from build123d import *

# Parameters (mm, degrees)
SKETCH1_W           = 16
SKETCH1_H           = 16
BOSS_EXTRUDE1_DEPTH = 1.5875
BOSS_EXTRUDE2_DEPTH = 3.625
BOSS_EXTRUDE3_DEPTH = 1.5875
SKETCH5_R           = 0.599365756
BOSS_EXTRUDE6_DEPTH = 50
SKETCH6_R           = 0.881021891
BOSS_EXTRUDE7_DEPTH = 2
BOSS_EXTRUDE8_DEPTH = 4
SKETCH8_R           = 1.431086417
BOSS_EXTRUDE9_DEPTH = 1.75
SKETCH9_R           = 1.026782917
SKETCH9_R_2         = 0.386874667
CUT_EXTRUDE1_DEPTH  = 0.5


with BuildPart() as part:
    # Sketch1 → Boss-Extrude1 (new body)
    with BuildSketch(Plane(origin=(0, 0, 0), x_dir=(1, 0, 0), z_dir=(0, 1, 0))):
        Rectangle(SKETCH1_W, SKETCH1_H)
    extrude(amount=BOSS_EXTRUDE1_DEPTH)

    # Sketch2 → Boss-Extrude2 (add)
    with BuildSketch(Plane(origin=(0, 1.5875, 0), x_dir=(1, 0, 0), z_dir=(0, 1, 0))):
        with BuildLine():
            Line((-6.5, -7.5), (6.5, -7.5))
            ThreePointArc((6.5, -7.5), (7.207106781, -7.207106781), (7.5, -6.5))
            Line((7.5, -6.5), (7.5, 6.5))
            ThreePointArc((7.5, 6.5), (7.207106781, 7.207106781), (6.5, 7.5))
            Line((6.5, 7.5), (-6.5, 7.5))
            ThreePointArc((-6.5, 7.5), (-7.207106781, 7.207106781), (-7.5, 6.5))
            Line((-7.5, 6.5), (-7.5, -6.5))
            ThreePointArc((-7.5, -6.5), (-7.207106781, -7.207106781), (-6.5, -7.5))
        make_face()
    extrude(amount=BOSS_EXTRUDE2_DEPTH)

    # Sketch4 → Boss-Extrude3 (add)
    with BuildSketch(Plane.XZ):
        Polygon((5, 6), (-5, 6), (-6, 5), (-6, -5), (-5, -6), (5, -6), (6, -5), (6, 5), align=None)
    extrude(amount=BOSS_EXTRUDE3_DEPTH)

    # Sketch5 → Boss-Extrude6 (add)
    with BuildSketch(Plane(origin=(6, 0, 0), x_dir=(0, 0, -1), z_dir=(1, 0, 0))):
        with Locations(Location((0, -0.711731406, 0), (0, 0, 180))):
            Circle(SKETCH5_R)
    extrude(amount=BOSS_EXTRUDE6_DEPTH)

    # Sketch6 → Boss-Extrude7 (add)
    with BuildSketch(Plane(origin=(56, 0, 0), x_dir=(0, 0, -1), z_dir=(1, 0, 0))):
        with Locations((0, -0.711731406)):
            Circle(SKETCH6_R)
    extrude(amount=BOSS_EXTRUDE7_DEPTH)

    # Sketch7 → Boss-Extrude8 (add)
    with BuildSketch(Plane(origin=(58, 0, 0), x_dir=(0, 0, -1), z_dir=(1, 0, 0))):
        with BuildLine():
            Line((-0.493950471, 0.22540454), (0.493950471, 0.22540454))
            ThreePointArc((0.493950471, 0.22540454), (1.431086417, -0.711731406), (0.493950471, -1.648867351))
            Line((0.493950471, -1.648867351), (-0.493950471, -1.648867351))
            ThreePointArc((-0.493950471, -1.648867351), (-1.431086417, -0.711731406), (-0.493950471, 0.22540454))
        make_face()
    extrude(amount=BOSS_EXTRUDE8_DEPTH)

    # Sketch8 → Boss-Extrude9 (add)
    with BuildSketch(Plane.XZ.offset(0.711731406)):
        with Locations(Location((60.568913583, 0, 0), (0, 0, 270))):
            Circle(SKETCH8_R)
    extrude(amount=BOSS_EXTRUDE9_DEPTH)

    # Sketch9 → Cut-Extrude1 (cut)
    with BuildSketch(Plane(origin=(0, -2.461731406, 0), x_dir=(-1, 0, 0), z_dir=(0, -1, 0))):
        with Locations(Location((-60.568913583, 0, 0), (0, 0, 90))):
            Circle(SKETCH9_R)
        with Locations(Location((-60.568913583, 0, 0), (0, 0, 90))):
            Circle(SKETCH9_R_2, mode=Mode.SUBTRACT)
    extrude(amount=-CUT_EXTRUDE1_DEPTH, mode=Mode.SUBTRACT)


solid = part.part
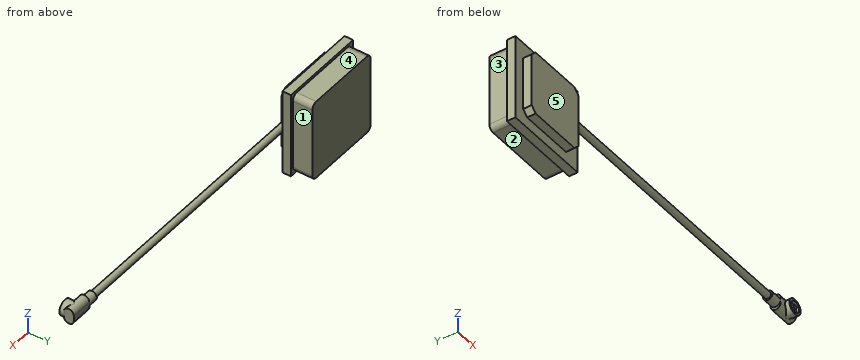
CAD build for the part. Positions are in the model's coordinates, mm. Face numbers are marked on the shaded views. A direction names the side the tool comes from. Coordinates: 2 decimals unless noted, no trailing zeros. Order: outer loops, then holes, each group sorted by start corner. A loop starts at its lowest first (then second) coordinate and runs counter-clockwise, first axis right, second up. Notation, with made-up numbers: (-4, 40) -> (48, 40) arc R15 ccw to (48, 51) -> close; hole circle Ø5 at (54, 37). An arc over 180 degrees is marked (long way). Answer in a Markdown table with one row per item.
1) Which spindle directions (+Z, -Z, +X, -X, +Y, -Y) get a long thin tool onto all of the face, cutting with end or side? Do the marked faces 1, 2, 3, 4 and 5. Say none if no direction does.
Check values:
| item | result |
|---|---|
| face 1 | +Z, -Z, +X, +Y |
| face 2 | -Z, +X, -X, +Y |
| face 3 | +Z, -Z, -X, +Y |
| face 4 | +Z, +X, -X, +Y |
| face 5 | +Z, -Z, -X, -Y |
2) Band-saw the part on B-B (x = 47.5). List the corners of the cut face in (y, z), and give its area (3 significant figures).
Check values:
| item | result |
|---|---|
| outline | circle Ø1.2 at (-0.71, 0) |
| area | 1.13 mm2 |
3) Band-saw the part on A-A (z = 3). List the corners of the cut face in (x, y), and give its area (3 significant figures).
Check values:
| item | result |
|---|---|
| outline | (-8, 0) -> (-6, 0) -> (-6, -1.59) -> (6, -1.59) -> (6, 0) -> (8, 0) -> (8, 1.59) -> (7.5, 1.59) -> (7.5, 5.21) -> (-7.5, 5.21) -> (-7.5, 1.59) -> (-8, 1.59) -> close |
| area | 98.8 mm2 |
4) Drill centre lines: line 1 (X direction, y = -2.3, z = 0); line 2 (Y direction, x = -3, z = 7.25); line 3 (Z direction, x = -1, y = 3.75). Where is each one in solid material? Low to high.
Check values:
| item | result |
|---|---|
| line 1 | 59.14 to 59.54, 60.18 to 60.96, 61.6 to 62 |
| line 2 | 0 to 5.21 |
| line 3 | -7.5 to 7.5 |
5) Flat gauge pins, fed straight in: P1, Ø1.8, axis at y = 3, z = 0.5, coming from the +X side; P2, Ø0.5, axis at x = -0.5, y = -1, coming from the +Z side; P3, Ø1.8, axis at y = 3.5, z = 2, coming from the -X side. Where does each tip first touch, or does it go through?
Check values:
| item | result |
|---|---|
| P1 | x = 7.5 |
| P2 | z = 6 |
| P3 | x = -7.5 |
